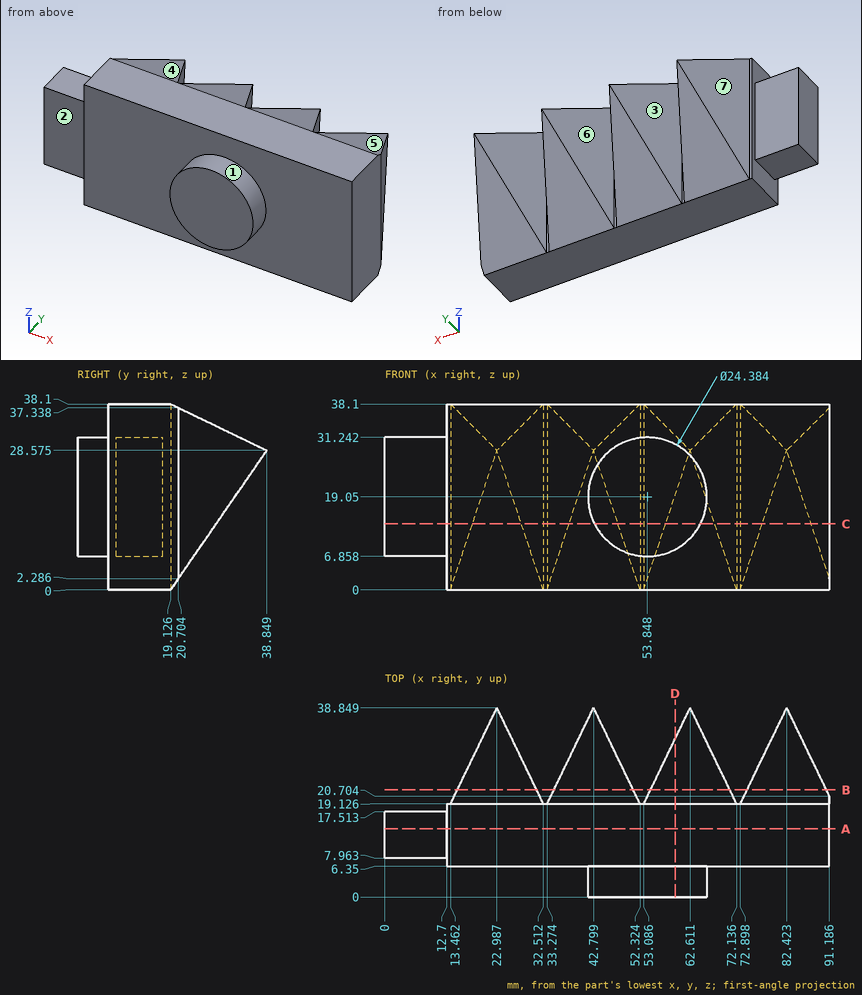
Source: three-view drawing plus pictorial views. Frame: mm from the lowest corner of the part. A direction names the side the tool comes from. Coordinates: 2 decimals unless noted, no trailing zeros. Write each loop counter-clockwise with the first axis right and the second up, starting at its lowest first coordinate (ties: lowest second). Pieces come first, ordered by that corner, then holes. Notation, with made-up numbers: (-7, 15.25) -> (33, 15.25) arc R27 ccw to (33, 48.25) -> close; hole circle Ø6 at (84, -14). An arc over 180 degrees is marked (long way). Write each question's results on one line, items separated by ' | '.
Item 1: Mould query, pull axis X, two halves, no side actions, for the marked faces 5, 6 and 7. Classes: +X half, -X half, draft (parallel to the pull), parting line (faces both ways), or undercut.
Conclusion:
face 5: draft | face 6: undercut | face 7: -X half
Item 2: Section query C-C on z = 13.5. Return loops of the section in (x, y), plus the area to 3 significant figures.
Conclusion:
outline: (0, 7.96) -> (12.7, 7.96) -> (12.7, 6.35) -> (42.99, 6.35) -> (42.99, 0) -> (64.7, 0) -> (64.7, 6.35) -> (91.19, 6.35) -> (91.19, 20.7) -> (87.45, 28.44) -> (77.4, 28.44) -> (72.9, 19.13) -> (72.14, 19.13) -> (67.64, 28.44) -> (57.59, 28.44) -> (53.09, 19.13) -> (52.32, 19.13) -> (47.82, 28.44) -> (37.77, 28.44) -> (33.27, 19.13) -> (32.51, 19.13) -> (28.01, 28.44) -> (17.96, 28.44) -> (13.46, 19.13) -> (12.7, 19.13) -> (12.7, 17.51) -> (0, 17.51) -> close | area: 1,800 mm^2
Item 3: Section query D-D on x = 59.5. Return loops of the section in (y, z), plus the area to 3 significant figures.
Conclusion:
outline: (0, 8.25) -> (6.35, 8.25) -> (6.35, 0) -> (19.13, 0) -> (32.41, 19.24) -> (32.41, 31.69) -> (19.13, 38.1) -> (6.35, 38.1) -> (6.35, 29.85) -> (0, 29.85) -> close | area: 960 mm^2
Item 4: Section query A-A on y = 14. Return loops of the section in (x, z), plus the area to 3 significant figures.
Conclusion:
outline: (0, 6.86) -> (12.7, 6.86) -> (12.7, 0) -> (91.19, 0) -> (91.19, 38.1) -> (12.7, 38.1) -> (12.7, 31.24) -> (0, 31.24) -> close | area: 3,300 mm^2
Item 5: Section query B-B on y = 22. Return loops of the section in (x, z), plus the area to 3 significant figures.
Conclusion:
outline: (14.85, 4.16) -> (31.12, 4.16) -> (31.12, 36.71) -> (14.85, 36.71) -> close; (34.66, 4.16) -> (50.94, 4.16) -> (50.94, 36.71) -> (34.66, 36.71) -> close; (54.47, 4.16) -> (70.75, 4.16) -> (70.75, 36.71) -> (54.47, 36.71) -> close; (74.29, 4.16) -> (90.56, 4.16) -> (90.56, 36.71) -> (74.29, 36.71) -> close | area: 2,120 mm^2
Item 6: Pin query (flat end, axial travel): pin 1 Ø14 at (x, z) = (6, 13.5) entering from -Y; pin 2 Ø4 at (x, z) = (30.5, 31.5) entering from +Y (1 decimal); pin 3 Ø1.5 at (x, y) = (16, 23) entering from -Z (1 decimal). Return the tip coordinate at first contact, or that it passes through.
Conclusion:
pin 1: stops at y = 6.35 | pin 2: stops at y = 27.4 | pin 3: stops at z = 4.5
Item 7: Set-up query: the marked faces 1, 2, 3 and 4. Return all of +Z, -Z, +X, -X, +Y, -Y with unobstructed straight access to the full face (end or side cutting, diameter ignored); none if empty.
Conclusion:
face 1: -Y | face 2: +Z, -Z, -X, -Y | face 3: +Z, -Z, +Y | face 4: +Z, +X, -X, +Y
Item 8: Material intervals for probe 1 along X at (y, z) = (33, 22.5) (1 decimal); probe 2 along X at (y, z) = (20, 29.5) (1 decimal); probe 3 along X at (y, z) = (10, 3.5), sorted ascending.
Conclusion:
probe 1: x = 20.2 to 25.8, 40 to 45.6, 59.8 to 65.4, 79.6 to 85.2 | probe 2: x = 13.9 to 32.1, 33.7 to 51.9, 53.5 to 71.7, 73.3 to 91.2 | probe 3: x = 12.7 to 91.19
